Geometry check sheet. Reference: the model listing, model coordinates, mm. Round coordinates to 2 decimals unless told otherwise and drop trailing zeros. Write each loop counter-clockwise with the first axis right and the second up, starting at its lowest first coordinate (ties: lowest second). Pieces come first, ordered by that corner, then holes. Notation, with made-up numbers: (-28.75, 23) - (-12.75, 23) arc R27 cw to (-12.75, 47) - close; hole circle Ø11 at (68.25, 3). An arc over 180 degrees is marked (long way). One line per question, with ' | ' between items. Start each with the question number.
from build123d import *


with BuildPart() as part:
    # Sweep1: sweep along a path in Sketch1
    with BuildLine(Plane(origin=(0, 0, 0), x_dir=(1, 0, 0), z_dir=(0, 1, 0))) as sweep1_path:
        Line((0, 0), (-90.078432584, 0))
        ThreePointArc((-90.078432584, 0), (-93.613966489, 0.645856533), (-96.692810861, 2.5))
        ThreePointArc((-96.692810861, 2.5), (-105, -1.25), (-96.692810861, -5))
        ThreePointArc((-96.692810861, -5), (-93.613966489, -3.145856533), (-90.078432584, -2.5))
        Line((-90.078432584, -2.5), (0, -2.5))
    # Sketch2 → Sweep1 (sweep)
    with BuildSketch(Plane(origin=(0, 0, 0), x_dir=(0, 0, -1), z_dir=(1, 0, 0))):
        with BuildLine():
            Line((0, -2.291287847), (0, 2.291287847))
            ThreePointArc((0, 2.291287847), (3.5, 0), (0, -2.291287847))
        make_face()
    sweep(path=sweep1_path.line)


solid = part.part
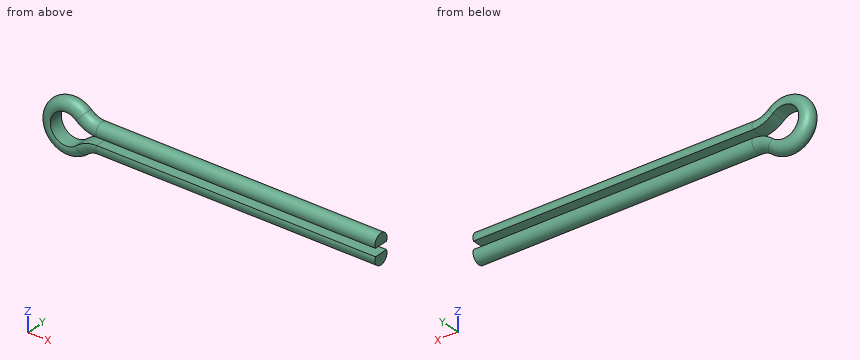
Q1. Go/stop test with flat-tipped pins: P1, Ø2.5, axis at x = -30, y = 0, coming from the -Z side; P2, Ø1, axis at y = -1.5, z = -0.5, coming from the -X side. Record where each tip stops, or that it passes through.
Q2. Thickness scan on line 1 (Z direction, x = -100, y = -0.2); line 2 (Y direction, x = -92, z = 4); line 3 (Z direction, x = -88.5, y = 1.25). Record the ranges inside material, lowest first.
Q3. Section check A-A, the plane x = -73. Record the cut outline in (y, z).
Q4. Section check B-B, the plane y = 0. Record the cut outline in (x, z) (3 decimals), then the cut area to 3 significant figures.
Result sheet:
1) P1: z = -3.5 | P2: x = -108.13
2) line 1: -7.24 to -3.75, 6.25 to 9.74 | line 2: -2.48 to 2.48 | line 3: -3.17 to 0, 2.5 to 5.67
3) outline: (-2.29, 0) arc R2.5 ccw (long way) to (2.29, 0) - close; (-2.29, 2.5) - (2.29, 2.5) arc R2.5 ccw (long way) to start
4) outline: (-96.693, -2.5) arc R5 cw (long way) to (-96.693, 5) arc R10 ccw to (-90.078, 2.5) - (0, 2.5) - (0, 6) - (-90.078, 6) arc R6.5 cw to (-94.378, 7.625) arc R8.5 ccw (long way) to (-94.378, -5.125) arc R6.5 cw to (-90.078, -3.5) - (0, -3.5) - (0, 0) - (-90.078, 0) arc R10 ccw to start | area: 781 mm²
